from build123d import *

# Parameters (mm, degrees)
SKETCH1_W                                           = 94
SKETCH1_H                                           = 68
BOSS_EXTRUDE1_DEPTH                                 = 10
M5_TAPPED_HOLE1_D                                   = 4.2
M5_TAPPED_HOLE1_DEPTH                               = 14
M5_TAPPED_HOLE1_TIP                                 = 1.2618073
SKETCH4_W                                           = 94
SKETCH4_H                                           = 32
CUT_EXTRUDE1_DEPTH                                  = 1
CHAMFER1_SIZE                                       = 3
CBORE_FOR_M4_HEX_SOCKET_HEAD_CAP_SCREW5_D           = 4.5
CBORE_FOR_M4_HEX_SOCKET_HEAD_CAP_SCREW5_CBORE_D     = 7.5
CBORE_FOR_M4_HEX_SOCKET_HEAD_CAP_SCREW5_CBORE_DEPTH = 5.8
M5_TAPPED_HOLE2_D                                   = 4.2
M5_TAPPED_HOLE2_DEPTH                               = 14
M5_TAPPED_HOLE2_TIP                                 = 1.2618073
M4_TAPPED_HOLE1_D                                   = 3.3
M4_TAPPED_HOLE1_DEPTH                               = 11.5
M4_TAPPED_HOLE1_TIP                                 = 0.991420021
CBORE_FOR_M4_HEX_SOCKET_HEAD_CAP_SCREW6_D           = 4.5
CBORE_FOR_M4_HEX_SOCKET_HEAD_CAP_SCREW6_CBORE_D     = 7.5
CBORE_FOR_M4_HEX_SOCKET_HEAD_CAP_SCREW6_CBORE_DEPTH = 5.8


with BuildPart() as part:
    # Sketch1 → Boss-Extrude1 (new body)
    with BuildSketch(Plane.XY):
        with Locations((47, 34)):
            Rectangle(SKETCH1_W, SKETCH1_H)
    extrude(amount=BOSS_EXTRUDE1_DEPTH)

    # M5 Tapped Hole1
    with Locations(Plane(origin=(9, 68, 5), x_dir=(1, 0, 0), z_dir=(0, 1, 0))):
        with Locations((0, 0), (20, 0), (56, 0), (76, 0)):
            Hole(M5_TAPPED_HOLE1_D / 2, depth=M5_TAPPED_HOLE1_DEPTH)
            with Locations((0, 0, -(M5_TAPPED_HOLE1_DEPTH + M5_TAPPED_HOLE1_TIP / 2))):  # 118° drill point
                Cone(0, M5_TAPPED_HOLE1_D / 2, M5_TAPPED_HOLE1_TIP, mode=Mode.SUBTRACT)

    # Sketch4 → Cut-Extrude1 (cut)
    with BuildSketch(Plane.XY.offset(10)):
        with Locations((47, 16)):
            Rectangle(SKETCH4_W, SKETCH4_H)
    extrude(amount=-CUT_EXTRUDE1_DEPTH, mode=Mode.SUBTRACT)

    # Chamfer1
    chamfer1_edges = [part.edges().sort_by_distance(p)[0] for p in [
        (0, 0, 4.5),
        (94, 0, 4.5),
    ]]
    chamfer(chamfer1_edges, length=CHAMFER1_SIZE)

    # CBORE for M4 Hex Socket Head Cap Screw5 (through all)
    with Locations(Plane(origin=(4, 17.7, 9), x_dir=(1, 0, 0), z_dir=(0, 0, 1))):
        with Locations((0, 0), (26, 0), (60, 0), (86, 0)):
            CounterBoreHole(CBORE_FOR_M4_HEX_SOCKET_HEAD_CAP_SCREW5_D / 2, CBORE_FOR_M4_HEX_SOCKET_HEAD_CAP_SCREW5_CBORE_D / 2, CBORE_FOR_M4_HEX_SOCKET_HEAD_CAP_SCREW5_CBORE_DEPTH)

    # M5 Tapped Hole2
    with Locations(Plane(origin=(7, 24.5, 9), x_dir=(1, 0, 0), z_dir=(0, 0, 1))):
        with Locations((0, 0), (0, -15), (80, 0), (80, -15)):
            Hole(M5_TAPPED_HOLE2_D / 2, depth=M5_TAPPED_HOLE2_DEPTH)
            with Locations((0, 0, -(M5_TAPPED_HOLE2_DEPTH + M5_TAPPED_HOLE2_TIP / 2))):  # 118° drill point
                Cone(0, M5_TAPPED_HOLE2_D / 2, M5_TAPPED_HOLE2_TIP, mode=Mode.SUBTRACT)

    # M4 Tapped Hole1
    with Locations(Plane(origin=(3.5, 61, 10), x_dir=(1, 0, 0), z_dir=(0, 0, 1))):
        with Locations((0, 0), (12, 0), (75, 0), (87, 0)):
            Hole(M4_TAPPED_HOLE1_D / 2, depth=M4_TAPPED_HOLE1_DEPTH)
            with Locations((0, 0, -(M4_TAPPED_HOLE1_DEPTH + M4_TAPPED_HOLE1_TIP / 2))):  # 118° drill point
                Cone(0, M4_TAPPED_HOLE1_D / 2, M4_TAPPED_HOLE1_TIP, mode=Mode.SUBTRACT)

    # CBORE for M4 Hex Socket Head Cap Screw6 (through all)
    with Locations(Plane(origin=(4, 43.7, 10), x_dir=(1, 0, 0), z_dir=(0, 0, 1))):
        with Locations((0, 0), (26, 0), (60, 0), (86, 0)):
            CounterBoreHole(CBORE_FOR_M4_HEX_SOCKET_HEAD_CAP_SCREW6_D / 2, CBORE_FOR_M4_HEX_SOCKET_HEAD_CAP_SCREW6_CBORE_D / 2, CBORE_FOR_M4_HEX_SOCKET_HEAD_CAP_SCREW6_CBORE_DEPTH)


solid = part.part
Model file for the job. Use its own axes, mm. A direction names the side the tool comes from. Give positions to 0.01 mm unless a question says otherwise; leave off trailing zeros. Loops run counter-clockwise (first coordinate to the right, second up) from the corner with the lowest first, then second, coordinate; pieces in that order, holes last.
1) Tool access for faces 4 (the cylindrical face through (3.512, 47.418, 7.141)), 5 (the conical face through (85.34, 52.96, 5.14)): list every direction of +Z, -Z, +X, -X, +Y, -Y with a clear straight run to the whole face (end or side of a thin tool).
2) Pull direction Z, two halves, no side cores. Call faces 1 (the cylindrical face through (93.577, 44.826, 7.141)), 2 (the conical face through (65.34, 52.96, 5.14)), 3 (the flat face through (46, 34, 0)): +Z half, -Z half, draft (parallel to the pull), parting line (faces both ways), or undercut.
3) Saw through at C-C (x = 78). Write the cut outline in (y, z), plus the area to 3 significant figures.
4) Flat gauge pins, fed straight in: pin 1 Ø2.5 at (x, y) = (30, 43.7) entering from +Z; pin 2 Ø7 at (x, y) = (64, 17.7) entering from +Z; pin 3 Ø9.5 at (x, y) = (39.5, 15) entering from +Z. Where does each tip first touch, or does it go through?
5) Saw through at B-B (y = 61). Count the separate pieces of the cut face and the enclosed holes in it, plus the area to 3 significant figures.
6) Saw through at A-A (y = 9.5). Write the cut outline in (x, z), plus the area to 3 significant figures.
7) Wall check: line 1 (X direction, y = 59, z = 5.25); line 2 (Y direction, x = 64, z = 8.45); line 3 (X direction, y = 57, z = 3.75). Give the ranges that are in metal, low to high.
Answer block:
1. face 4: +Z
1. face 5: +Y
2. face 1: draft
2. face 2: undercut
2. face 3: -Z half
3. outline: (0, 0) - (59.43, 0) - (59.43, 10) - (32, 10) - (32, 9) - (0, 9) - close; (62.57, 0) - (68, 0) - (68, 10) - (62.57, 10) - close
3. area: 617 mm2
4. pin 1: passes through
4. pin 2: stops at z = 3.2
4. pin 3: stops at z = 9
5. separate pieces: 5
5. enclosed holes: 4
5. area: 753 mm2
6. outline: (0, 0) - (4.9, 0) - (4.9, 9) - (0, 9) - close; (9.1, 0) - (84.9, 0) - (84.9, 9) - (9.1, 9) - close; (89.1, 0) - (94, 0) - (94, 9) - (89.1, 9) - close
6. area: 770 mm2
7. line 1: x = 0 to 6.91, 11.09 to 26.91, 31.09 to 62.91, 67.09 to 82.91, 87.09 to 94
7. line 2: y = 0 to 13.95, 21.45 to 39.95, 47.45 to 68
7. line 3: x = 0 to 7.31, 10.69 to 27.31, 30.69 to 63.31, 66.69 to 83.31, 86.69 to 94
